Could you check a few things on this model? Use its own coordinates, in mm. Round coordinates to 2 decimals unless told otherwise and drop trailing zeros. Order: outer loops, then holes, each group sorted by start corner. A loop starts at its lowest first (then second) coordinate and runs counter-clockwise, first axis right, second up.
Autodesk Inventor part; units mm, degrees
ref_plane "YZ Plane" through (0, 0, 0) normal (1, 0, 0) x (0, 1, 0)
ref_plane "XZ Plane" through (0, 0, 0) normal (0, 1, 0) x (-1, 0, 0)
ref_plane "XY Plane" through (0, 0, 0) normal (0, 0, 1) x (1, 0, 0)
sketch "Sketch1" plane through (0, 0, 0) normal (0, 0, 1) x (1, 0, 0)
  line L0 (-60, 7.5) -> (60, 7.5)
  line L1 (60, 7.5) -> (60, -7.5)
  line L2 (60, -7.5) -> (-60, -7.5)
  line L3 (-60, -7.5) -> (-60, 7.5)
  line L4 (-60, 7.5) -> (60, -7.5) construction
  line L5 (60, 7.5) -> (-60, -7.5) construction
  circle A0 centre (-52.5, 0) radius 2.5
  circle A1 centre (52.5, 0) radius 2.5
  point P0 (0, 0)
  point P1 (-60, 0)
  point P2 (60, 0)
  dimension "d0" = 120
  dimension "d1" = 15
  dimension "d2" = 5
  dimension "d3" = 7.5
  dimension "d4" = 7.5
extrude "Extrusion1" add sketch "Sketch1" along normal blind 3
sketch "Sketch2" plane through (0, 0, 3) normal (0, 0, 1) x (1, 0, 0)
  line L0 (-40, 0) -> (40, 0) construction
  point P0 (0, 0)
  point P1 (0, 0)
  dimension "d7" = 80
hole "Hole1" at (-40, 0, 3) at (40, 0, 3) direction (0, 0, -1) diameter 3.3 depth 36.25 countersink diameter 6.5 countersink angle 90
fillet "Fillet1" radius 2 4 edges at (-60, 7.5, 1.5) (-60, -7.5, 1.5) (60, 7.5, 1.5) (60, -7.5, 1.5)
equation "\"d4\" = d3"
properties part number "Power Supply Wall Mount v1"
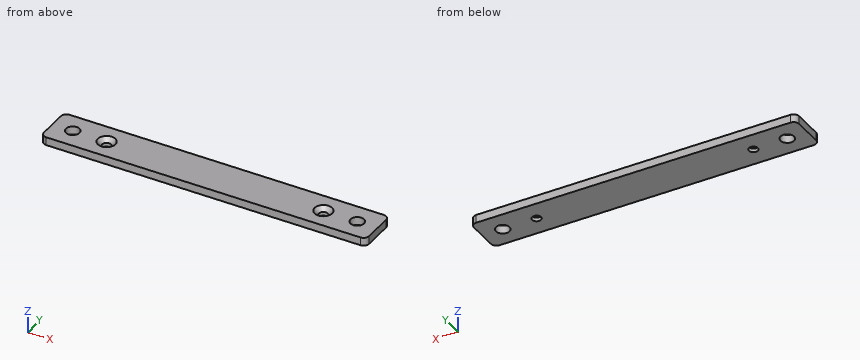
Q1. Imagine slicing it at A-A, the plane y = 0. Please give me the cut outline in (x, z), then the cut area to 3 significant figures.
Q2. Imagine slicing it at B-B, the plane z = 2.25. Please give me the cut outline in (x, y), then the cut area to 3 significant figures.
Q3. Imagine slicing it at D-D, the plane x = -40. Please give me the cut outline in (y, z).
Q4. Imagine slicing it at C-C, the plane x = -52.5. Please give me the cut outline in (y, z).
Q5. I need wall thicknesses on L1, parallel to Y at x = -40, z = 1; L2, parallel to X at y = 1.25, z = 2.75; L3, parallel to Y at x = 52.5, z = 2.35. Which ranges of each line are inside material? Lowest first, please.
Filled in:
1. outline: (-60, 0) - (-55, 0) - (-55, 3) - (-60, 3) - close; (-50, 0) - (-41.65, 0) - (-41.65, 1.4) - (-43.25, 3) - (-50, 3) - close; (-38.35, 0) - (38.35, 0) - (38.35, 1.4) - (36.75, 3) - (-36.75, 3) - (-38.35, 1.4) - close; (41.65, 0) - (50, 0) - (50, 3) - (43.25, 3) - (41.65, 1.4) - close; (55, 0) - (60, 0) - (60, 3) - (55, 3) - close
1. area: 305 mm2
2. outline: (-60, -5.5) arc R2 ccw to (-58, -7.5) - (58, -7.5) arc R2 ccw to (60, -5.5) - (60, 5.5) arc R2 ccw to (58, 7.5) - (-58, 7.5) arc R2 ccw to (-60, 5.5) - close; hole circle Ø5 at (-52.5, 0); hole circle Ø5 at (-40, 0); hole circle Ø5 at (40, 0); hole circle Ø5 at (52.5, 0)
2. area: 1,720 mm2
3. outline: (-7.5, 0) - (-1.65, 0) - (-1.65, 1.4) - (-3.25, 3) - (-7.5, 3) - close; (1.65, 0) - (7.5, 0) - (7.5, 3) - (3.25, 3) - (1.65, 1.4) - close
4. outline: (-7.5, 0) - (-2.5, 0) - (-2.5, 3) - (-7.5, 3) - close; (2.5, 0) - (7.5, 0) - (7.5, 3) - (2.5, 3) - close
5. L1: y = -7.5 to -1.65, 1.65 to 7.5
5. L2: x = -60 to -54.67, -50.33 to -42.73, -37.27 to 37.27, 42.73 to 50.33, 54.67 to 60
5. L3: y = -7.5 to -2.5, 2.5 to 7.5
